from build123d import *

# Parameters (mm, degrees)
CROQUIS1_R              = 31.5
CROQUIS1_R_2            = 1.5
SALIENTE_EXTRUIR1_DEPTH = 3
CORTAR_EXTRUIR2_DEPTH   = 1.5
CROQUIS4_R              = 2.5
CORTAR_EXTRUIR3_DEPTH   = 3
CROQUIS5_W              = 3
CROQUIS5_H              = 15
SALIENTE_EXTRUIR2_DEPTH = 25
CORTAR_EXTRUIR4_START   = -9
CROQUIS6_R              = 2.7
CORTAR_EXTRUIR4_DEPTH   = 9
CORTAR_EXTRUIR5_DEPTH   = 2


with BuildPart() as part:
    # Croquis1 → Saliente-Extruir1 (new body)
    with BuildSketch(Plane.XY):
        with Locations((-43.449193048, 8.207110309)):
            Circle(CROQUIS1_R)
        with Locations((-60.066202406, 24.824119667)):
            Circle(CROQUIS1_R_2, mode=Mode.SUBTRACT)
        with Locations((-26.83218369, 24.824119667)):
            Circle(CROQUIS1_R_2, mode=Mode.SUBTRACT)
        with Locations((-26.83218369, -8.409899049)):
            Circle(CROQUIS1_R_2, mode=Mode.SUBTRACT)
        with Locations((-60.066202406, -8.409899049)):
            Circle(CROQUIS1_R_2, mode=Mode.SUBTRACT)
    extrude(amount=SALIENTE_EXTRUIR1_DEPTH)

    # Croquis3 → Cortar-Extruir2 (cut)
    with BuildSketch(Plane.XY.offset(3)):
        with BuildLine():
            Line((-41.199193048, 22.957110309), (-40.349193048, 10.457110309))
            Line((-40.349193048, 10.457110309), (-36.699193048, 10.457110309))
            ThreePointArc((-36.699193048, 10.457110309), (-34.449193048, 8.207110309), (-36.699193048, 5.957110309))
            Line((-36.699193048, 5.957110309), (-39.699193048, 5.957110309))
            Line((-39.699193048, 5.957110309), (-41.199193048, -8.542889691))
            ThreePointArc((-41.199193048, -8.542889691), (-43.449193048, -10.792889691), (-45.699193048, -8.542889691))
            Line((-45.699193048, -8.542889691), (-47.199193048, 5.957110309))
            Line((-47.199193048, 5.957110309), (-50.199193048, 5.957110309))
            ThreePointArc((-50.199193048, 5.957110309), (-52.449193048, 8.207110309), (-50.199193048, 10.457110309))
            Line((-50.199193048, 10.457110309), (-46.549193048, 10.457110309))
            Line((-46.549193048, 10.457110309), (-45.699193048, 22.957110309))
            ThreePointArc((-45.699193048, 22.957110309), (-43.449193048, 25.207110309), (-41.199193048, 22.957110309))
        make_face()
    extrude(amount=-CORTAR_EXTRUIR2_DEPTH, mode=Mode.SUBTRACT)

    # Croquis4 → Cortar-Extruir3 (cut)
    with BuildSketch(Plane(origin=(0, 0, 0), x_dir=(-1, 0, 0), z_dir=(0, 0, -1))):
        with Locations((43.449193048, 8.207110309)):
            Circle(CROQUIS4_R)
    extrude(amount=-CORTAR_EXTRUIR3_DEPTH, mode=Mode.SUBTRACT)

    # Croquis5 → Saliente-Extruir2 (add)
    with BuildSketch(Plane(origin=(0, 0, 0), x_dir=(-1, 0, 0), z_dir=(0, 0, -1))):
        with Locations((40.449193048, 27.207110309)):
            Rectangle(CROQUIS5_W, CROQUIS5_H)
        with Locations((46.449193048, 27.207110309)):
            Rectangle(CROQUIS5_W, CROQUIS5_H)
    extrude(amount=SALIENTE_EXTRUIR2_DEPTH)

    # Croquis6 → Cortar-Extruir4 (cut)
    with BuildSketch(Plane(origin=(-38.949193048, 0, 0), x_dir=(0, 0, -1), z_dir=(1, 0, 0)).offset(CORTAR_EXTRUIR4_START)):
        with BuildLine():
            Line((25, 34.707110309), (17.5, 34.707110309))
            ThreePointArc((17.5, 34.707110309), (22.803300859, 32.510411168), (25, 27.207110309))
            Line((25, 27.207110309), (25, 34.707110309))
        make_face()
        with BuildLine():
            Line((25, 19.707110309), (25, 27.207110309))
            ThreePointArc((25, 27.207110309), (22.803300859, 21.90380945), (17.5, 19.707110309))
            Line((17.5, 19.707110309), (25, 19.707110309))
        make_face()
        with Locations(Location((17.5, 27.207110309, 0), (0, 0, 90))):
            Circle(CROQUIS6_R)
    extrude(amount=CORTAR_EXTRUIR4_DEPTH, mode=Mode.SUBTRACT)

    # Croquis7 → Cortar-Extruir5 (cut)
    with BuildSketch(Plane(origin=(0, 0, 0), x_dir=(-1, 0, 0), z_dir=(0, 0, -1))):
        Polygon((30.065345197, 24.824119667), (28.448764443, 27.624119667), (25.215602936, 27.624119667), (23.599022182, 24.824119667), (25.215602936, 22.024119667), (28.448764443, 22.024119667), align=None)
        Polygon((63.299363913, 24.824119667), (61.682783159, 27.624119667), (58.449621652, 27.624119667), (56.833040898, 24.824119667), (58.449621652, 22.024119667), (61.682783159, 22.024119667), align=None)
        Polygon((30.065345197, -8.409899049), (28.448764443, -5.609899049), (25.215602936, -5.609899049), (23.599022182, -8.409899049), (25.215602936, -11.209899049), (28.448764443, -11.209899049), align=None)
        Polygon((56.833040898, -8.409899049), (58.449621652, -11.209899049), (61.682783159, -11.209899049), (63.299363913, -8.409899049), (61.682783159, -5.609899049), (58.449621652, -5.609899049), align=None)
    extrude(amount=-CORTAR_EXTRUIR5_DEPTH, mode=Mode.SUBTRACT)


solid = part.part
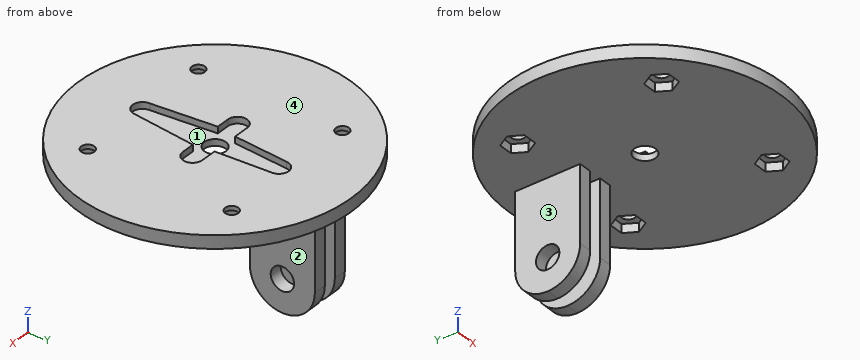
The listing builds one solid part. Answer for the finished solid, in the listing's coordinates (mm). Face numbers are marked on the shaded views. A direction names the side the tool comes from. Coordinates: 2 decimals unless noted, no trailing zeros. Order: outer loops, then holes, each group sorted by start corner. A loop starts at its lowest first (then second) coordinate and runs counter-clockwise, first axis right, second up.
Q1. A cutting plane is placed at D-D, the plane z = -19. Write down the section's boundary in (x, y).
Q2. A cutting plane is placed at A-A, the plane z = -14. Write down the section's boundary in (x, y), and give its area (3 significant figures).
Q3. Given P1, Ø2.5, axis at x = -46, z = -5.5, coming from the +Y side; P2, Ø1.6, axis at x = -59.5, z = 1, coming from the -Y side; P3, Ø5, axis at x = -49, z = -5, coming from the -Y side; P4, Ø12, axis at y = -15.5, z = -10, coming from the -X side, each flat-ended and moving along its own axis, determine where each tip first touches the part or whether it passes through.
Q4. A cutting plane is placed at B-B, the plane x = -27. Write down the section's boundary in (y, z), and give its area (3 significant figures).
Q5. Consider line 1 (Y direction, x = -39.8, z = -17.5); line 2 (X direction, y = 24.5, z = -3); line 3 (Z direction, x = -54, y = -13). Determine where each line is inside the solid, lowest interval first.
Q6. For a pull along Y with two mould halves and no side action, classify the marked faces 1 and 2 as pulls with the +Y half, pulls with the -Y half, needs draft (parallel to the pull), parting line crosses it, or undercut.
Q7. Which of the six approach directions +Z, -Z, +X, -X, +Y, -Y give full straight-line access (tool end or side, diameter ignored) to the marked faces 3 and 4?
Q8. A cutting plane is placed at C-C, the plane y = -4. Write down the section's boundary in (x, z), and give its area (3 significant figures).
Answers follow:
1. outline: (-47.95, 19.86) - (-44.95, 19.86) - (-44.95, 24.96) - (-47.95, 24.96) - close; (-47.95, 29.45) - (-44.95, 29.45) - (-44.95, 34.56) - (-47.95, 34.56) - close; (-41.95, 19.86) - (-38.95, 19.86) - (-38.95, 24.96) - (-41.95, 24.96) - close; (-41.95, 29.45) - (-38.95, 29.45) - (-38.95, 34.56) - (-41.95, 34.56) - close
2. outline: (-47.95, 19.71) - (-44.95, 19.71) - (-44.95, 34.71) - (-47.95, 34.71) - close; (-41.95, 19.71) - (-38.95, 19.71) - (-38.95, 34.71) - (-41.95, 34.71) - close
2. area: 90.0 mm2
3. P1: stops at y = 34.71
3. P2: stops at y = -19.35
3. P3: stops at y = 19.71
3. P4: passes through
4. outline: (-18.66, 0) - (-11.21, 0) - (-11.21, 2) - (-9.9, 2) - (-9.9, 3) - (-18.66, 3) - close; (-6.92, 2) - (-5.61, 2) - (-5.61, 0) - (22.02, 0) - (22.02, 2) - (23.33, 2) - (23.33, 3) - (-6.92, 3) - close; (26.31, 2) - (27.62, 2) - (27.62, 0) - (35.07, 0) - (35.07, 3) - (26.31, 3) - close
4. area: 133 mm2
5. line 1: y = 19.71 to 24.51, 29.91 to 34.71
5. line 2: x = -47.95 to -44.95, -41.95 to -38.95
5. line 3: z = 0 to 3
6. face 1: undercut
6. face 2: needs draft
7. face 3: -Z, -X, +Y, -Y
7. face 4: +Z, +X, -X, +Y, -Y
8. outline: (-72.49, 0) - (-14.41, 0) - (-14.41, 3) - (-40.73, 3) - (-40.73, 1.5) - (-46.17, 1.5) - (-46.17, 3) - (-72.49, 3) - close
8. area: 166 mm2
